Could you check a few things on this model? Use its own coordinates, in mm. A direction names the side the tool comes from. Coordinates: 2 decimals unless noted, no trailing zeros. Write each loop counter-clockwise with the first axis right and the second up, starting at its lowest first coordinate (ties: lowest second). Pieces come first, ordered by that corner, then holes. Notation, with made-up numbers: (25.5, 35.25) - (33.5, 35.25) arc R10 cw to (33.5, 50.25) - close; hole circle Ø1 at (7.25, 57). An arc over 180 degrees is marked (long way). Write item = value, one per line. Start each with the question number.
```python
from build123d import *

# Parameters (mm, degrees)
PAD_DEPTH    = 3
SKETCH001_R  = 1.5
PAD001_DEPTH = 6
SKETCH002_R  = 2.1
POCKET_DEPTH = 2
SKETCH003_R  = 3
PAD002_DEPTH = 3
FILLET_R     = 2.75


with BuildPart() as part:
    # Sketch → Pad (new body)
    with BuildSketch(Plane.XY):
        Polygon((-9.25, -33), (14.25, -33), (14.25, -11.5), (7, -11.5), (7, 33), (4, 33), (4, 43), (-4, 43), (-4, 33), (-7, 33), (-7, -11.5), (-9.25, -11.5), align=None)
    extrude(amount=PAD_DEPTH)

    # Sketch001 → Pad001 (join, symmetric)
    with BuildSketch(Plane.YZ):
        with Locations((40, 1.5)):
            Circle(SKETCH001_R)
    extrude(amount=PAD001_DEPTH, both=True)

    # Sketch002 (on Face5 of Pad001) → Pocket (cut)
    with BuildSketch(Plane.XY.offset(3)):
        with Locations((2.5, -23)):
            Circle(SKETCH002_R)
    extrude(amount=-POCKET_DEPTH, mode=Mode.SUBTRACT)

    # Sketch003 (on Face5 of Pocket) → Pad002 (join)
    with BuildSketch(Plane.XY.offset(3)):
        with Locations((0, 23)):
            Circle(SKETCH003_R)
    extrude(amount=PAD002_DEPTH)

    # Fillet
    fillet_edges = [part.edges().sort_by_distance(p)[0] for p in [
        (-3, 23, 6),
    ]]
    fillet(fillet_edges, radius=FILLET_R)


solid = part.part
```
1) Suppose I cut it at D-D on x = 9.75. Please give me the cut outline in (y, z), plus the area to 3 significant figures.
2) Suppose I cut it at B-B on y = -23. Please give me the cut outline in (x, z), plus the area to 3 significant figures.
3) Which directions (+Z, -Z, +X, -X, +Y, -Y) give clear straight access to the entire face, cutting with the end or side of a thin tool? Please do faces 1 (the flat face through (-6, 40, 2)), 2 (the flat face through (2, -23, 1)), 3 (the flat face through (7, 10, 1)), 4 (the flat face through (6, 33, 1)).
4) Suppose I cut it at A-A on x = -5. Please give me the cut outline in (y, z), plus the area to 3 significant figures.
5) For P1, Ø1.5, axis at y = 35, z = 1, coming from the +X side; P2, Ø1.5, axis at y = 40.5, z = 2, coming from the +X side; P3, Ø1.5, axis at x = 5.5, z = 2, coming from the +Y side; P4, Ø12, axis at x = -6, y = 20, coming from the -Z side, each with a flat end and sliding along its axis, tell me the tip position at first contact or that it passes through.
6) If I drill on probe 1 along Y at (x, z) = (2.5, 2.2); probe 2 along Z at (x, y) = (-5.25, 12.5); probe 3 along Y at (x, z) = (9.5, 1.85), over which ranges is the centre line in solid material (lowest first)? Write a range as [from, to].
7) Thinking about a two-plate mould opening in Y: for faces 5 (the flat face through (-4, 36, 1)), 6 (the flat face through (-5, 33, 1)), 7 (the flat face through (-8, -11.5, 1)), 8 (the flat face through (-9.25, -22, 1)), which applies, +Y half, -Y half, draft (parallel to the pull), parting line (faces both ways), or undercut?
8) Suppose I cut it at C-C on z = 2.3. Please give me the cut outline in (x, y).
Reply:
q1.outline = (-33, 0) - (-11.5, 0) - (-11.5, 3) - (-33, 3) - close
q1.area = 64.5 mm^2
q2.outline = (-9.25, 0) - (14.25, 0) - (14.25, 3) - (4.6, 3) - (4.6, 1) - (0.4, 1) - (0.4, 3) - (-9.25, 3) - close
q2.area = 62.1 mm^2
q3.face_1 = +Z, -Z, -X, +Y
q3.face_2 = +Z
q3.face_3 = +Z, -Z, +X, +Y
q3.face_4 = +Z, -Z, +X
q4.outline = (-33, 0) - (33, 0) - (33, 3) - (-33, 3) - close; circle Ø3 at (40, 1.5)
q4.area = 205 mm^2
q5.P1 = 4
q5.P2 = 6
q5.P3 = 41.5
q5.P4 = 0
q6.probe_1 = [-33, -25.1], [-20.9, 43]
q6.probe_2 = [0, 3]
q6.probe_3 = [-33, -11.5]
q7.face_5 = undercut
q7.face_6 = undercut
q7.face_7 = +Y half
q7.face_8 = draft
q8.outline = (-9.25, -33) - (14.25, -33) - (14.25, -11.5) - (7, -11.5) - (7, 33) - (4, 33) - (4, 38.73) - (6, 38.73) - (6, 41.27) - (4, 41.27) - (4, 43) - (-4, 43) - (-4, 41.27) - (-6, 41.27) - (-6, 38.73) - (-4, 38.73) - (-4, 33) - (-7, 33) - (-7, -11.5) - (-9.25, -11.5) - close; hole circle Ø4.2 at (2.5, -23)
